Model file for the job. Use its own axes, mm. Face numbers are marked on the shaded views. A direction names the side the tool comes from. Coordinates: 2 decimals unless noted, no trailing zeros. Write each loop counter-clockwise with the first axis right and the second up, starting at its lowest first coordinate (ties: lowest second). Pieces come first, ordered by that corner, then holes.
Q1. Band-saw the part on C-C, the plane y = 0. Write the cut outline in (x, z), plus the area to 4 significant figures.
Q2. Pin check, flat tips, straight feed: P1, Ø5, axis at y = 16.5, z = 4.5, coming from the -X side; P2, Ø8, axis at y = 10.5, z = 4.5, coming from the +X side; P3, Ø3, axis at y = -5, z = 13, coming from the +X side; P4, Ø14, axis at x = -18, y = -6.5, coming from the +Z side. Stop position of each tip, or through.
Q3. Which spindle directions (+Z, -Z, +X, -X, +Y, -Y) get a long thin tool onto all of the face, cutting with end or side? Do the marked faces 1, 2 and 3. Say none if no direction does.
Q4. Band-saw the part on B-B, the plane z = 7.5. Write the cut outline in (x, y).
Q5. Band-saw the part on A-A, the plane x = 0. Write the cut outline in (y, z).
Q6. Band-saw the part on D-D, the plane z = 23.25. Write the cut outline in (x, y).
Q7. Drill centre lines: probe 1 along Y at (x, z) = (0, 7.25); probe 2 along Y at (x, z) = (0, 11); probe 3 along X at (y, z) = (16, 7). Where is each one in solid material? Low to high.
Q8. Pull direction Y, two halves, no side cores. Call the marked faces 4, 5 and 6: released by +Y, released by -Y, zero draft, split by the parting line, or undercut.
from build123d import *

# Parameters (mm, degrees)
SKETCH_1_R      = 32.5
SKETCH_1_R_2    = 25.5
EXTRUDE_1_DEPTH = 25
EXTRUDE_2_DEPTH = 10
SKETCH_2_3_R    = 5
SKETCH_2_3_R_2  = 2.75
EXTRUDE_3_DEPTH = 25


with BuildPart() as part:
    # Sketch 1 → Extrude 1 (new body)
    with BuildSketch(Plane.XY):
        Circle(SKETCH_1_R)
        Circle(SKETCH_1_R_2, mode=Mode.SUBTRACT)
    extrude(amount=EXTRUDE_1_DEPTH)

    # Sketch 2 → Extrude 2 (add)
    with BuildSketch(Plane.XY):
        with BuildLine():
            Line((-1.5, 25.455844123), (-1.5, 4.769696007))
            ThreePointArc((-1.5, 4.769696007), (-0.758788496, 4.942088629), (0, 5))
            Line((0, 5), (0, 25.5))
            ThreePointArc((0, 25.5), (-0.750324887, 25.48895864), (-1.5, 25.455844123))
        make_face()
        with BuildLine():
            Line((0, 25.5), (0, 5))
            ThreePointArc((0, 5), (0.758788496, 4.942088629), (1.5, 4.769696007))
            Line((1.5, 4.769696007), (1.5, 25.455844123))
            ThreePointArc((1.5, 25.455844123), (0.750324887, 25.48895864), (0, 25.5))
        make_face()
        with BuildLine():
            ThreePointArc((-3.38067791, -3.683886109), (-4.330127019, -2.5), (-4.88067791, -1.085809898))
            Line((-4.88067791, -1.085809898), (-22.795407685, -11.428883956))
            ThreePointArc((-22.795407685, -11.428883956), (-22.083647797, -12.75), (-21.295407685, -14.026960167))
            Line((-21.295407685, -14.026960167), (-3.38067791, -3.683886109))
        make_face()
        with BuildLine():
            ThreePointArc((4.88067791, -1.085809898), (4.330127019, -2.5), (3.38067791, -3.683886109))
            Line((3.38067791, -3.683886109), (21.295407685, -14.026960167))
            ThreePointArc((21.295407685, -14.026960167), (22.083647797, -12.75), (22.795407685, -11.428883956))
            Line((22.795407685, -11.428883956), (4.88067791, -1.085809898))
        make_face()
    extrude(amount=EXTRUDE_2_DEPTH)

    # Sketch 2_3 → Extrude 3 (add)
    with BuildSketch(Plane.XY):
        with Locations(Location((0, 0, 0), (0, 0, 192.542396876))):
            Circle(SKETCH_2_3_R)
        Circle(SKETCH_2_3_R_2, mode=Mode.SUBTRACT)
    extrude(amount=EXTRUDE_3_DEPTH)


solid = part.part
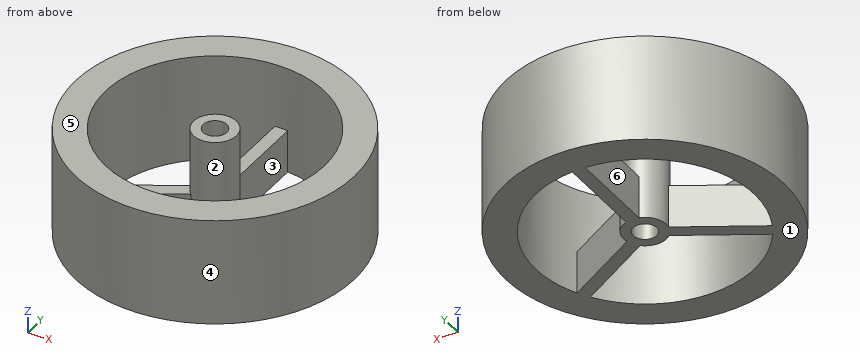
Answer sheet:
1. outline: (-32.5, 0) - (-25.5, 0) - (-25.5, 25) - (-32.5, 25) - close; (-5, 0) - (-2.75, 0) - (-2.75, 25) - (-5, 25) - close; (2.75, 0) - (5, 0) - (5, 25) - (2.75, 25) - close; (25.5, 0) - (32.5, 0) - (32.5, 25) - (25.5, 25) - close
1. area: 462.5 mm2
2. P1: stops at x = -29.33
2. P2: stops at x = 31.84
2. P3: stops at x = 32.31
2. P4: stops at z = 25
3. face 1: -Z, +X, -X, +Y, -Y
3. face 2: +Z
3. face 3: +Z, -Z
4. outline: circle Ø65 at (0, 0); hole (-22.8, -11.43) - (-4.88, -1.09) arc R5 cw to (-1.5, 4.77) - (-1.5, 25.46) arc R25.5 ccw to start; hole (-21.3, -14.03) arc R25.5 ccw to (21.3, -14.03) - (3.38, -3.68) arc R5 cw to (-3.38, -3.68) - close; hole circle Ø5.5 at (0, 0); hole (1.5, 4.77) arc R5 cw to (4.88, -1.09) - (22.8, -11.43) arc R25.5 ccw to (1.5, 25.46) - close
5. outline: (-32.5, 0) - (-25.5, 0) - (-25.5, 25) - (-32.5, 25) - close; (-5, 0) - (-2.75, 0) - (-2.75, 25) - (-5, 25) - close; (2.75, 0) - (32.5, 0) - (32.5, 25) - (25.5, 25) - (25.5, 10) - (5, 10) - (5, 25) - (2.75, 25) - close
6. outline: circle Ø65 at (0, 0); circle Ø10 at (0, 0); hole circle Ø51 at (0, 0); hole circle Ø5.5 at (0, 0)
7. probe 1: y = -32.5 to -25.5, -5 to -2.75, 2.75 to 32.5
7. probe 2: y = -32.5 to -25.5, -5 to -2.75, 2.75 to 5, 25.5 to 32.5
7. probe 3: x = -28.29 to -19.86, -1.5 to 1.5, 19.86 to 28.29
8. face 4: split by the parting line
8. face 5: zero draft
8. face 6: undercut
